Here's how the part is built. I have some questions about the finished solid (model axes, mm). Face numbers are marked on the shaded views. A direction names the side the tool comes from. Round coordinates to 2 decimals unless told otherwise and drop trailing zeros. Loops run counter-clockwise (first coordinate to the right, second up) from the corner with the lowest first, then second, coordinate; pieces in that order, holes last. Notation, with made-up numbers: M 25,66 L 67,66 A19 cw 67,92 Z; hole C -22.75,58.25 d5. An arc over 180 degrees is marked long. Use a Markdown table: item, result.
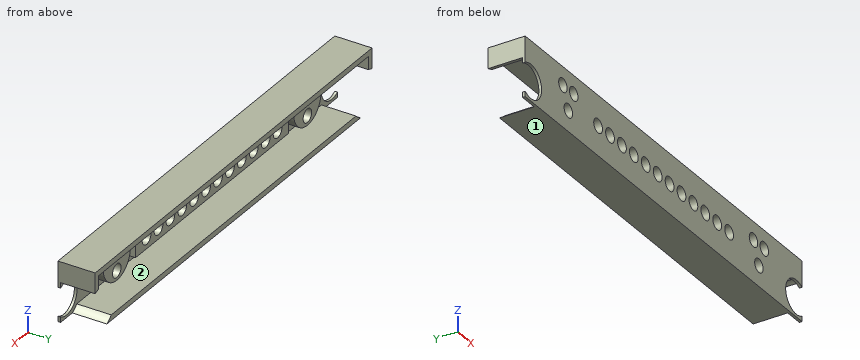
```python
from build123d import *

# Parameters (mm, degrees)
SKETCH1_W           = 162.7
SKETCH1_H           = 22
BOSS_EXTRUDE1_DEPTH = 13.75
SKETCH2_W           = 158.7
SKETCH2_H           = 18
CUT_EXTRUDE1_DEPTH  = 12.75
SKETCH4_W           = 90
SKETCH4_H           = 8.5
BOSS_EXTRUDE2_DEPTH = 5.8
SKETCH3_R           = 2.575
CUT_EXTRUDE2_DEPTH  = 84.233917365
SKETCH7_R           = 8
CUT_EXTRUDE4_DEPTH  = 12.75
SKETCH5_R           = 6.25
CUT_EXTRUDE5_DEPTH  = 84.233917365
SKETCH8_R           = 8
BOSS_EXTRUDE4_DEPTH = 4.8
SKETCH10_W          = 90
SKETCH10_H          = 8.5
CUT_EXTRUDE6_DEPTH  = 1
SKETCH11_R          = 2.5
CUT_EXTRUDE7_DEPTH  = 83.474389964


with BuildPart() as part:
    # Sketch1 → Boss-Extrude1 (new body)
    with BuildSketch(Plane(origin=(0, 0, 0), x_dir=(1, 0, 0), z_dir=(0, 1, 0))):
        Rectangle(SKETCH1_W, SKETCH1_H)
    extrude(amount=BOSS_EXTRUDE1_DEPTH)

    # Sketch2 → Cut-Extrude1 (cut)
    with BuildSketch(Plane(origin=(0, 13.75, 0), x_dir=(1, 0, 0), z_dir=(0, 1, 0))):
        Rectangle(SKETCH2_W, SKETCH2_H)
    extrude(amount=-CUT_EXTRUDE1_DEPTH, mode=Mode.SUBTRACT)

    # Sketch4 → Boss-Extrude2 (add)
    with BuildSketch(Plane(origin=(0, 1, 0), x_dir=(1, 0, 0), z_dir=(0, 1, 0))):
        Rectangle(SKETCH4_W, SKETCH4_H)
    extrude(amount=BOSS_EXTRUDE2_DEPTH)

    # Sketch3 → Cut-Extrude2 (cut, through all)
    with BuildSketch(Plane.XZ):
        with Locations(Location((-3.5, -0.1, 0), (0, 0, 270))):
            Circle(SKETCH3_R)
        with Locations(Location((-10.5, -0.1, 0), (0, 0, 270))):
            Circle(SKETCH3_R)
        with Locations(Location((-17.5, -0.1, 0), (0, 0, 270))):
            Circle(SKETCH3_R)
        with Locations(Location((-24.5, -0.1, 0), (0, 0, 270))):
            Circle(SKETCH3_R)
        with Locations(Location((-31.5, -0.1, 0), (0, 0, 270))):
            Circle(SKETCH3_R)
        with Locations(Location((-38.5, -0.1, 0), (0, 0, 270))):
            Circle(SKETCH3_R)
        with Locations(Location((38.5, -0.1, 0), (0, 0, 270))):
            Circle(SKETCH3_R)
        with Locations(Location((31.5, -0.1, 0), (0, 0, 270))):
            Circle(SKETCH3_R)
        with Locations(Location((24.5, -0.1, 0), (0, 0, 270))):
            Circle(SKETCH3_R)
        with Locations(Location((17.5, -0.1, 0), (0, 0, 270))):
            Circle(SKETCH3_R)
        with Locations(Location((10.5, -0.1, 0), (0, 0, 270))):
            Circle(SKETCH3_R)
        with Locations(Location((3.5, -0.1, 0), (0, 0, 270))):
            Circle(SKETCH3_R)
    extrude(amount=-CUT_EXTRUDE2_DEPTH, mode=Mode.SUBTRACT)

    # Sketch7 → Cut-Extrude4 (cut)
    with BuildSketch(Plane(origin=(0, 13.75, 0), x_dir=(1, 0, 0), z_dir=(0, 1, 0))):
        with Locations((-77.98, 3.8)):
            Circle(SKETCH7_R)
        with Locations((77.98, 3.8)):
            Circle(SKETCH7_R)
    extrude(amount=-CUT_EXTRUDE4_DEPTH, mode=Mode.SUBTRACT)

    # Sketch5 → Cut-Extrude5 (cut, through all)
    with BuildSketch(Plane.XZ):
        with Locations((-77.98, -3.8)):
            Circle(SKETCH5_R)
        with Locations((77.98, -3.8)):
            Circle(SKETCH5_R)
    extrude(amount=-CUT_EXTRUDE5_DEPTH, mode=Mode.SUBTRACT)

    # Sketch8 → Boss-Extrude4 (add)
    with BuildSketch(Plane(origin=(0, 1, 0), x_dir=(1, 0, 0), z_dir=(0, 1, 0))):
        with Locations((-56, -1.1)):
            Circle(SKETCH8_R)
        with Locations((56, -1.1)):
            Circle(SKETCH8_R)
    extrude(amount=BOSS_EXTRUDE4_DEPTH)

    # Sketch10 → Cut-Extrude6 (cut)
    with BuildSketch(Plane(origin=(0, 6.8, 0), x_dir=(1, 0, 0), z_dir=(0, 1, 0))):
        Rectangle(SKETCH10_W, SKETCH10_H)
    extrude(amount=-CUT_EXTRUDE6_DEPTH, mode=Mode.SUBTRACT)

    # Sketch11 → Cut-Extrude7 (cut, through all)
    with BuildSketch(Plane(origin=(0, 5.8, 0), x_dir=(1, 0, 0), z_dir=(0, 1, 0))):
        with Locations(Location((-56, 3.4, 0), (0, 0, 270))):
            Circle(SKETCH11_R)
        with Locations(Location((-59.181980515, -4.281980515, 0), (0, 0, 270))):
            Circle(SKETCH11_R)
        with Locations(Location((-52.818019485, -4.281980515, 0), (0, 0, 270))):
            Circle(SKETCH11_R)
        with Locations(Location((52.818019485, -4.281980515, 0), (0, 0, 90))):
            Circle(SKETCH11_R)
        with Locations(Location((59.181980515, -4.281980515, 0), (0, 0, 90))):
            Circle(SKETCH11_R)
        with Locations(Location((56, 3.4, 0), (0, 0, 90))):
            Circle(SKETCH11_R)
    extrude(amount=-CUT_EXTRUDE7_DEPTH, mode=Mode.SUBTRACT)


solid = part.part
```
Q1. For the marked faces 1 and 2, which set-ups out of +Z, -Z, +X, -X, +Y, -Y let a thin tool reach every point of the face, with its end or its side?
Return value:
| item | result |
|---|---|
| face 1 | -Z, +X, -X, +Y, -Y |
| face 2 | +X, -X, +Y |
Q2. Will these pins go through, and if not, where does the flat tip stop? P1, Ø10, axis at x = -34.5, z = -2, coming from the +Y side; P2, Ø1, axis at x = 1, z = -5, coming from the +Y side; P3, Ø1.5, axis at y = 5, z = 2.5, coming from the -X side.
Return value:
| item | result |
|---|---|
| P1 | stops at y = 5.8 |
| P2 | stops at y = 1 |
| P3 | stops at x = -63.97 |
Q3. I need wall thicknesses on line 1 (Z direction, x = 34, y = 11.5); line 2 (X direction, y = 12.25, z = 5.5); line 3 (Z direction, x = -50, y = 1.5). Which ranges of each line are inside material? Lowest first, please. Write a range as from..to.
Return value:
| item | result |
|---|---|
| line 1 | z = -11..-9, 9..11 |
| line 2 | x = -81.35..-79.35, 79.35..81.35 |
| line 3 | z = -11..-9, -4.19..6.39, 9..11 |
Q4. Imagine slicing it at A-A, the plane y = 10.75. Please give me the cut outline in (x, z), then the cut area to 3 significant figures.
Return value:
| item | result |
|---|---|
| outline | M -81.35,3.46 A8 cw -79.35,4.08 L -79.35,9 L 79.35,9 L 79.35,4.08 A8 cw 81.35,3.46 L 81.35,11 L -81.35,11 Z; M -74.49,-11 L 74.49,-11 A8 cw 71.9,-9 L -71.9,-9 A8 cw Z |
| area | 638 mm^2 |
Q5. Imagine slicing it at B-B, the plane x = 38.5. Please give me the cut outline in (y, z) (3 decimals).
Return value:
| item | result |
|---|---|
| outline | M 0,-11 L 13.75,-11 L 13.75,-9 L 1,-9 L 1,-4.25 L 5.8,-4.25 L 5.8,-2.675 L 0,-2.675 Z; M 0,2.475 L 5.8,2.475 L 5.8,4.25 L 1,4.25 L 1,9 L 13.75,9 L 13.75,11 L 0,11 Z |
